from build123d import *

# Parameters (mm, degrees)
SKETCH1_R           = 1.5875
BOSS_EXTRUDE1_DEPTH = 17.8816
SKETCH2_R           = 4.0015
BOSS_EXTRUDE2_DEPTH = 11.8872


with BuildPart() as part:
    # Sketch1 → Boss-Extrude1 (new body)
    with BuildSketch(Plane.XY):
        Circle(SKETCH1_R)
    extrude(amount=-BOSS_EXTRUDE1_DEPTH)

    # Sketch2 → Boss-Extrude2 (add)
    with BuildSketch(Plane.XY.offset(-2.9972)):
        Circle(SKETCH2_R)
    extrude(amount=-BOSS_EXTRUDE2_DEPTH)


solid = part.part
Geometry check sheet. Reference: the model listing, model coordinates, mm. A direction names the side the tool comes from. Give positions to 0.01 mm unless a question says otherwise; leave off trailing zeros. Order: outer loops, then holes, each group sorted by start corner. A loop starts at its lowest first (then second) coordinate and runs counter-clockwise, first axis right, second up. Notation, with made-up numbers: M -24.75,86.25 L -16.75,86.25 A25 cw -16.75,120.25 Z; hole C -11.5,18.25 d1. An arc over 180 degrees is marked long. Use a Markdown table: item, result.
Item 1: Section check A-A (x = 0). Record the cut outline in (y, z).
Answers follow:
| item | result |
|---|---|
| outline | M -4,-14.88 L -1.59,-14.88 L -1.59,-17.88 L 1.59,-17.88 L 1.59,-14.88 L 4,-14.88 L 4,-3 L 1.59,-3 L 1.59,0 L -1.59,0 L -1.59,-3 L -4,-3 Z |
Item 2: Depth check by flat-ended pin: P1, Ø1.5, axis at x = -2, z = -3, coming from the -Y side; P2, Ø1.5, axis at x = 3, z = -13.5, coming from the +Y side; P3, Ø1, axis at y = 1, z = -7, coming from the +X side. Enter the tip coordinate at first touch or a pass-through.
Answers follow:
| item | result |
|---|---|
| P1 | stops at y = -3.8 |
| P2 | stops at y = 3.31 |
| P3 | stops at x = 3.97 |
Item 3: Material ranges on line 1 along Z through (x, y) = (-2.25, -1.5); line 2 along Y through (x, z) = (0, -16); line 3 along Y through (x, z) = (1, -14), recorded low to high.
Answers follow:
| item | result |
|---|---|
| line 1 | z = -14.88 to -3 |
| line 2 | y = -1.59 to 1.59 |
| line 3 | y = -3.87 to 3.87 |
Item 4: Section check D-D (x = 3). Record the cut outline in (y, z).
Answers follow:
| item | result |
|---|---|
| outline | M -2.65,-14.88 L 2.65,-14.88 L 2.65,-3 L -2.65,-3 Z |
Item 5: Section check C-C (z = -16.25). Record the cut outline in (x, y) (1 decimal), and give its area (3 significant figures).
Answers follow:
| item | result |
|---|---|
| outline | C 0,0 d3.2 |
| area | 7.92 mm2 |
Item 6: Tool access check on faces 1 (the cylindrical face through (-0.34, -1.55, -1.48)), 2 (the flat face through (0, 0, -17.882)), 3 (the cylindrical face through (-0.34, -1.55, -16.36)). Record the directions out of +Z, -Z, +X, -X, +Y, -Y that give a thin tool (end or side, any length) a straight path to the whole face; none if there is none.
Answers follow:
| item | result |
|---|---|
| face 1 | +Z |
| face 2 | -Z, +X, -X, +Y, -Y |
| face 3 | -Z |
